Geometry: see drawing. Coordinates: mm, zero at the bounding-box minimum. A direction names the side the tool comes from. Coordinates: 2 decimals unless noted, no trailing zeros. Write each loop counter-clockwise with the first axis right and the second up, starting at its lowest first coordinate (ties: lowest second). Pieces come first, ordered by that corner, then holes. Notation, with made-up numbers: (-5, -21) -> (4, -21) arc R23 cw to (4, -9) -> close; hole circle Ø9 at (32, 8.25). An arc over 180 degrees is marked (long way). Use one line per item in the form item = value. Start each with the question number.
(1) Cut plane C-C on y = 24.5. Return the cut outline in (x, z), plus the area to 3 significant figures.
(2) Cut plane A-A on z = 17.5. Return the cut outline in (x, y), plus the area to 3 significant figures.
(3) Ray query, line 1 along X through (y, z) = (9.5, 14.5); line 2 along Y through (x, z) = (25, 27); line 3 along Z through (x, y) = (125, 50). Return the intervals inside material, ascending.
(4) First-contact query: pin 1 (1 mm diameter, centred on x = 15, y = 10.5, fed in from -Z); pin 2 (24 mm diameter, centred on x = 124, y = 27, fed in from +Z). Flat tips, straight axial feed; report the tip coordinate or a pass-through.
(5) Cut plane B-B on x = 25.4. Return the cut outline in (y, z).
(6) Cut plane D-D on y = 46.5. Return the cut outline in (x, z).
(7) Set-up query: the marked faces 1, 2, 3 and 4. Return all of +Z, -Z, +X, -X, +Y, -Y with unobstructed straight access to the full face (end or side cutting, diameter ignored); none if empty.
(8) Pull-direction query (Y, two-part tool) for the marked faces 5, 6 and 7; classes: released by +Y, released by -Y, zero draft, split by the parting line, or undercut.
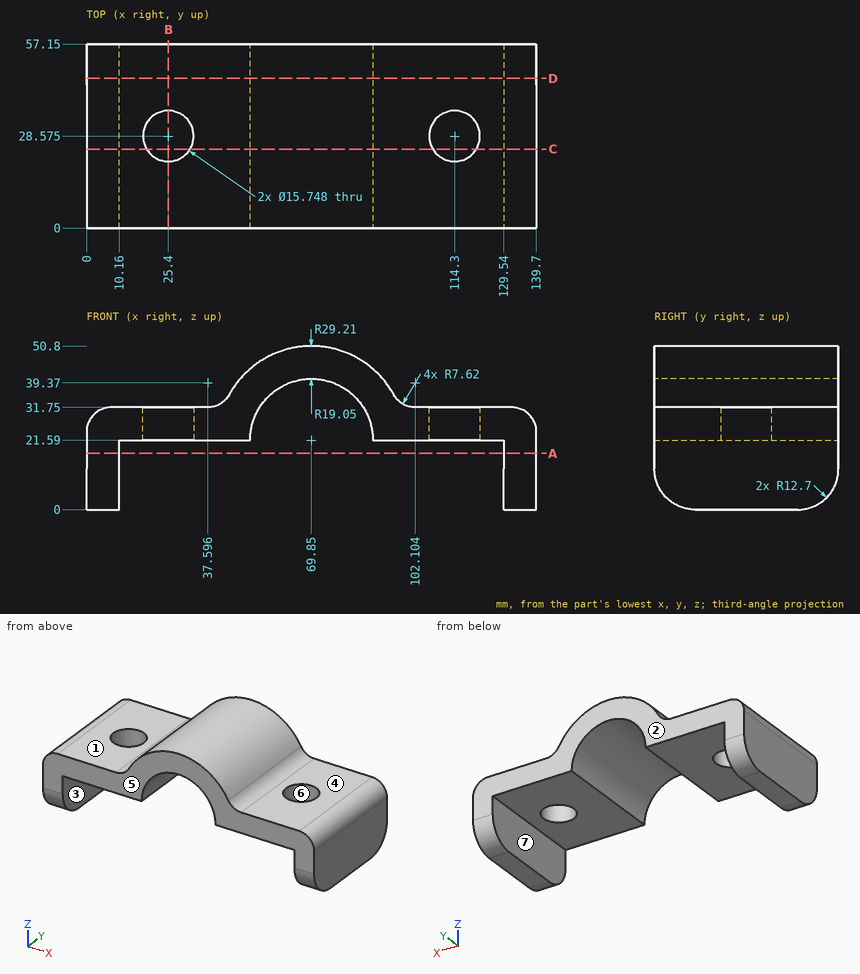
Values:
q1.outline = (0, 0) -> (10.16, 0) -> (10.16, 21.59) -> (18.66, 21.59) -> (18.66, 31.75) -> (7.62, 31.75) arc R7.62 ccw to (0, 24.13) -> close; (32.14, 21.59) -> (50.8, 21.59) arc R19.05 cw to (88.9, 21.59) -> (107.56, 21.59) -> (107.56, 31.75) -> (102.1, 31.75) arc R7.62 cw to (95.43, 35.69) arc R29.21 ccw to (44.27, 35.69) arc R7.62 cw to (37.6, 31.75) -> (32.14, 31.75) -> close; (121.04, 21.59) -> (129.54, 21.59) -> (129.54, 0) -> (139.7, 0) -> (139.7, 24.13) arc R7.62 ccw to (132.08, 31.75) -> (121.04, 31.75) -> close
q1.area = 1,760 mm2
q2.outline = (0, 0) -> (10.16, 0) -> (10.16, 57.15) -> (0, 57.15) -> close; (129.54, 0) -> (139.7, 0) -> (139.7, 57.15) -> (129.54, 57.15) -> close
q2.area = 1,160 mm2
q3.line_1 = 0 to 10.16, 129.54 to 139.7
q3.line_2 = 0 to 20.71, 36.44 to 57.15
q3.line_3 = 21.59 to 31.75
q4.pin_1 = 21.59
q4.pin_2 = 31.75
q5.outline = (0, 21.59) -> (20.7, 21.59) -> (20.7, 31.75) -> (0, 31.75) -> close; (36.45, 21.59) -> (57.15, 21.59) -> (57.15, 31.75) -> (36.45, 31.75) -> close
q6.outline = (0, 0.17) -> (10.16, 0.17) -> (10.16, 21.59) -> (50.8, 21.59) arc R19.05 cw to (88.9, 21.59) -> (129.54, 21.59) -> (129.54, 0.17) -> (139.7, 0.17) -> (139.7, 24.13) arc R7.62 ccw to (132.08, 31.75) -> (102.1, 31.75) arc R7.62 cw to (95.43, 35.69) arc R29.21 ccw to (44.27, 35.69) arc R7.62 cw to (37.6, 31.75) -> (7.62, 31.75) arc R7.62 ccw to (0, 24.13) -> close
q7.face_1 = +Z, -X, +Y, -Y
q7.face_2 = +Z, -Z, +X, -X, +Y
q7.face_3 = -Z, +Y, -Y
q7.face_4 = +Z, +X, +Y, -Y
q8.face_5 = released by -Y
q8.face_6 = undercut
q8.face_7 = zero draft
